```python
from build123d import *

# Parameters (mm, degrees)
BOSS_EXTRUDE1_OUTLINE_R   = 228.6
BOSS_EXTRUDE1_OUTLINE_R_2 = 2.0701
BOSS_EXTRUDE1_DEPTH       = 3.175
SKETCH3_W                 = 283.8196
SKETCH3_H                 = 182.2196
SKETCH3_R                 = 2.0701
CUT_EXTRUDE1_DEPTH        = 324.304810705
FILLET1_R                 = 3.175
CUT_EXTRUDE2_DEPTH        = 324.304810705
FILLET2_R                 = 9.525


# Read off the part's stored shape, not the designer's step: Boss-Extrude1
with BuildPart() as part:
    # Boss-Extrude1 outline → Boss-Extrude1 (new body)
    with BuildSketch(Plane(origin=(0, 0, 0), x_dir=(1, 0, 0), z_dir=(0, 1, 0))):
        Circle(BOSS_EXTRUDE1_OUTLINE_R)
        with Locations((-157.935764401, -157.935764401)):
            Circle(BOSS_EXTRUDE1_OUTLINE_R_2, mode=Mode.SUBTRACT)
        with Locations((-144.46538022, -144.46538022)):
            Circle(BOSS_EXTRUDE1_OUTLINE_R_2, mode=Mode.SUBTRACT)
        with Locations((0, -223.3549)):
            Circle(BOSS_EXTRUDE1_OUTLINE_R_2, mode=Mode.SUBTRACT)
        with Locations((0, -204.3049)):
            Circle(BOSS_EXTRUDE1_OUTLINE_R_2, mode=Mode.SUBTRACT)
        with Locations((157.935764401, -157.935764401)):
            Circle(BOSS_EXTRUDE1_OUTLINE_R_2, mode=Mode.SUBTRACT)
        with Locations((144.46538022, -144.46538022)):
            Circle(BOSS_EXTRUDE1_OUTLINE_R_2, mode=Mode.SUBTRACT)
        with Locations((-223.3549, 0)):
            Circle(BOSS_EXTRUDE1_OUTLINE_R_2, mode=Mode.SUBTRACT)
        with Locations((-204.3049, 0)):
            Circle(BOSS_EXTRUDE1_OUTLINE_R_2, mode=Mode.SUBTRACT)
        with Locations((-144.46538022, 144.46538022)):
            Circle(BOSS_EXTRUDE1_OUTLINE_R_2, mode=Mode.SUBTRACT)
        with Locations((-157.935764401, 157.935764401)):
            Circle(BOSS_EXTRUDE1_OUTLINE_R_2, mode=Mode.SUBTRACT)
        with Locations((204.3049, 0)):
            Circle(BOSS_EXTRUDE1_OUTLINE_R_2, mode=Mode.SUBTRACT)
        with Locations((223.3549, 0)):
            Circle(BOSS_EXTRUDE1_OUTLINE_R_2, mode=Mode.SUBTRACT)
        with Locations((0, 204.3049)):
            Circle(BOSS_EXTRUDE1_OUTLINE_R_2, mode=Mode.SUBTRACT)
        with Locations((0, 223.3549)):
            Circle(BOSS_EXTRUDE1_OUTLINE_R_2, mode=Mode.SUBTRACT)
        with Locations((144.46538022, 144.46538022)):
            Circle(BOSS_EXTRUDE1_OUTLINE_R_2, mode=Mode.SUBTRACT)
        with Locations((157.935764401, 157.935764401)):
            Circle(BOSS_EXTRUDE1_OUTLINE_R_2, mode=Mode.SUBTRACT)
    extrude(amount=BOSS_EXTRUDE1_DEPTH)

    # Sketch3 → Cut-Extrude1 (cut, through all)
    with BuildSketch(Plane.XZ):
        Rectangle(SKETCH3_W, SKETCH3_H)
        with Locations(Location((147.1549, -96.3549, 0), (0, 0, 270))):
            Circle(SKETCH3_R)
        with Locations(Location((56.0451, -96.3549, 0), (0, 0, 270))):
            Circle(SKETCH3_R)
        with Locations(Location((45.5549, -96.3549, 0), (0, 0, 90))):
            Circle(SKETCH3_R)
        with Locations(Location((-45.5549, -96.3549, 0), (0, 0, 90))):
            Circle(SKETCH3_R)
        with Locations(Location((-56.0451, -96.3549, 0), (0, 0, 270))):
            Circle(SKETCH3_R)
        with Locations(Location((-147.1549, -96.3549, 0), (0, 0, 270))):
            Circle(SKETCH3_R)
        with Locations(Location((-147.1549, 96.3549, 0), (0, 0, 90))):
            Circle(SKETCH3_R)
        with Locations(Location((-56.0451, 96.3549, 0), (0, 0, 90))):
            Circle(SKETCH3_R)
        with Locations(Location((-45.5549, 96.3549, 0), (0, 0, 270))):
            Circle(SKETCH3_R)
        with Locations(Location((45.5549, 96.3549, 0), (0, 0, 270))):
            Circle(SKETCH3_R)
        with Locations(Location((56.0451, 96.3549, 0), (0, 0, 90))):
            Circle(SKETCH3_R)
        with Locations(Location((147.1549, 96.3549, 0), (0, 0, 90))):
            Circle(SKETCH3_R)
    extrude(amount=-CUT_EXTRUDE1_DEPTH, mode=Mode.SUBTRACT)

    # Fillet1
    fillet1_edges = [part.edges().sort_by_distance(p)[0] for p in [
        (-141.9098, 1.5875, -91.1098),
        (-141.9098, 1.5875, 91.1098),
        (141.9098, 1.5875, 91.1098),
        (141.9098, 1.5875, -91.1098),
    ]]
    fillet(fillet1_edges, radius=FILLET1_R)

    # Sketch4 → Cut-Extrude2 (cut, through all)
    with BuildSketch(Plane.XZ):
        with BuildLine():
            Line((-9.525, -195.653083917), (-9.525, -101.6))
            Line((-9.525, -101.6), (-167.476251663, -101.6))
            ThreePointArc((-167.476251663, -101.6), (-100.219042208, -168.306263846), (-9.525, -195.653083917))
        make_face()
        with BuildLine():
            Line((167.476251663, -101.6), (9.525, -101.6))
            Line((9.525, -101.6), (9.525, -195.653083917))
            ThreePointArc((9.525, -195.653083917), (100.219042208, -168.306263846), (167.476251663, -101.6))
        make_face()
        with BuildLine():
            Line((9.525, 101.6), (167.476251663, 101.6))
            ThreePointArc((167.476251663, 101.6), (100.219042208, 168.306263846), (9.525, 195.653083917))
            Line((9.525, 195.653083917), (9.525, 101.6))
        make_face()
        with BuildLine():
            ThreePointArc((-9.525, 195.653083917), (-100.219042208, 168.306263846), (-167.476251663, 101.6))
            Line((-167.476251663, 101.6), (-9.525, 101.6))
            Line((-9.525, 101.6), (-9.525, 195.653083917))
        make_face()
    extrude(amount=-CUT_EXTRUDE2_DEPTH, mode=Mode.SUBTRACT)

    # Fillet2
    fillet2_edges = [part.edges().sort_by_distance(p)[0] for p in [
        (-167.476251663, 1.5875, -101.6),
        (-9.525, 1.5875, -101.6),
        (-9.525, 1.5875, -195.653083917),
        (9.525, 1.5875, -195.653083917),
        (9.525, 1.5875, -101.6),
        (167.476251663, 1.5875, -101.6),
        (167.476251663, 1.5875, 101.6),
        (9.525, 1.5875, 101.6),
        (9.525, 1.5875, 195.653083917),
        (-9.525, 1.5875, 195.653083917),
        (-9.525, 1.5875, 101.6),
        (-167.476251663, 1.5875, 101.6),
    ]]
    fillet(fillet2_edges, radius=FILLET2_R)


solid = part.part
```
Work out the finished part from the listing and answer in its coordinate system (mm). A direction names the side the tool comes from. Coordinates: 2 decimals unless noted, no trailing zeros. Loops run counter-clockwise (first coordinate to the right, second up) from the corner with the lowest first, then second, coordinate; pieces in that order, holes last.
1) Consider probe 1 along X at (y, z) = (1.9, 0) (3 decimals); probe 2 along Z at (x, y) = (-6, 2.3); probe 3 along Z at (x, y) = (136.5, 1.05). Determine where each line is inside the solid, lowest interval first.
Results:
probe 1: x = -228.6 to -225.425, -221.285 to -206.375, -202.235 to -141.91, 141.91 to 202.235, 206.375 to 221.285, 225.425 to 228.6
probe 2: z = -228.52 to -91.11, 91.11 to 228.52
probe 3: z = -183.37 to -140.49, -101.6 to -91.11, 91.11 to 101.6, 140.49 to 183.37
2) For a pull along X with two mould halves and no side action, classify faces 1 (the cylindrical face through (97.84, 1.57, 169.7)), 2 (the flat face through (-3, 0, 98)), 3 (the cylindrical face through (-228.38, 1.57, -10.05)) as +X half, -X half, draft (parallel to the pull), parting line (faces both ways), or undercut.
Results:
face 1: undercut
face 2: draft
face 3: parting line
3) Section B-B (z = 69) is taken. Give the vertices of the cut face in (x, y) (3 decimals).
Results:
outline: (-217.938, 0) - (-141.91, 0) - (-141.91, 3.175) - (-217.938, 3.175) - close; (141.91, 0) - (217.938, 0) - (217.938, 3.175) - (141.91, 3.175) - close
4) Flat-ended cylindrical pins translate along their axes: pin 1 (1 mm diameter, centred on x = -94, y = 1.5, fed in from -Z); pin 2 (6.5 mm diameter, centred on x = -45.55, z = -96.35, fed in from +Y) (3 decimals); pin 3 (1.6 mm diameter, centred on x = -11, y = 1, fed in from +Z); pin 4 (1 mm diameter, centred on y = 0.5, z = 64.5, fed in from +X). Find the tip coordinate at first contact, or state that the pin passes through.
Results:
pin 1: stops at z = -208.6
pin 2: stops at y = 3.175
pin 3: stops at z = 228.37
pin 4: stops at x = 219.46
5) Section A-A (x = -128) is taken. Give the vertices of the cut face in (y, z) (3 decimals).
Results:
outline: (0, -189.404) - (3.175, -189.404) - (3.175, -148.28) - (0, -148.28) - close; (0, -101.6) - (3.175, -101.6) - (3.175, -91.11) - (0, -91.11) - close; (0, 91.11) - (3.175, 91.11) - (3.175, 101.6) - (0, 101.6) - close; (0, 148.28) - (3.175, 148.28) - (3.175, 189.404) - (0, 189.404) - close
6) Section D-D (y = 0.5) is taken. Give the number of separate pieces and of enclosed holes in the cut face, plus the area to 3 significant figures.
Results:
separate pieces: 1
enclosed holes: 33
area: 71,500 mm2
7) Section C-C (z = -55) is taken. Give the vertices of the cut face in (x, y) (3 decimals).
Results:
outline: (-221.885, 0) - (-141.91, 0) - (-141.91, 3.175) - (-221.885, 3.175) - close; (141.91, 0) - (221.885, 0) - (221.885, 3.175) - (141.91, 3.175) - close
8) For faces 4 (the flat face through (-3, 3.175, 98)), 5 (the cylindrical face through (95.858, 1.565, -170.828)), determine the directions among +Z, -Z, +X, -X, +Y, -Y from which every point of the face is accessible in a straight line to the end or side of a thin tool.
Results:
face 4: +Z, -Z, +X, -X, +Y
face 5: +Y, -Y
